```python
from build123d import *

# Parameters (mm, degrees)
F0_W      = 10
F0_H      = 79
F1_DEPTH  = 10
F2_W      = 10
F2_H      = 2
F3_DEPTH  = 15
F4_W      = 10
F4_H      = 2
F5_DEPTH  = 30
F7_DEPTH  = 10.001
F8_R      = 0.99999
F9_W      = 4.9229283333
F9_H      = 15
F10_DEPTH = 7


# Not quite as in the source:
# - a fillet or chamfer is up to 0.001 mm smaller than in the source, because OpenCascade refuses the exact size


with BuildPart() as f1:
    # F0 (on Top) → F1 (new body)
    with BuildSketch(Plane.XY):
        Rectangle(F0_W, F0_H)
    extrude(amount=F1_DEPTH)

    # F2 (on face) → F3 (join)
    with BuildSketch(Plane.XY.offset(10)):
        with Locations((0, -38.5)):
            Rectangle(F2_W, F2_H)
    extrude(amount=F3_DEPTH)

    # F4 (on face) → F5 (join)
    with BuildSketch(Plane.XY.offset(10)):
        with Locations((0, 38.5)):
            Rectangle(F4_W, F4_H)
    extrude(amount=F5_DEPTH)

    # F6 (on face) → F7 (cut, through all)
    with BuildSketch(Plane.YZ.offset(5)):
        Polygon((34.5, 5), (-43.3395786217, 0), (34.5, 0), align=None)
    extrude(amount=-F7_DEPTH, mode=Mode.SUBTRACT)

    # F8 (radius 1 in the source; OpenCascade refuses exactly that, so slightly less here)
    f8_edges = [f1.edges().sort_by_distance(p)[0] for p in [
        (0, -39.5, 25),
        (0, -37.5, 25),
        (0, 37.5, 40),
        (0, 39.5, 40),
        (0, -37.5, 10),
        (0, 37.5, 10),
    ]]
    fillet(f8_edges, radius=F8_R)

    # F9 (on face) → F10 (cut)
    with BuildSketch(Plane.YZ.offset(5)):
        with Locations((-37.0385358334, 17.5)):
            Rectangle(F9_W, F9_H)
    extrude(amount=-F10_DEPTH, mode=Mode.SUBTRACT)


solid = f1.part
```
Geometry check sheet. Reference: the model listing, model coordinates, mm. A direction names the side the tool comes from. Round coordinates to 2 decimals unless told otherwise and drop trailing zeros. Order: outer loops, then holes, each group sorted by start corner. A loop starts at its lowest first (then second) coordinate and runs counter-clockwise, first axis right, second up. Notation, with made-up numbers: (-40, 38) - (-12, 38) arc R20 cw to (-12, 69) - close; hole circle Ø3 at (-38.75, -25.75). An arc over 180 degrees is marked (long way). Use a Markdown table: item, result. Add a question column.
(1) Tool access check on faces 1 (the flat face through (-2, -39, 18)), 2 (the flat face through (0.07, -1.982, 2.657)), 3 (the flat face through (0, 37, 0)), 4 (the flat face through (0, 37.5, 25)), 5 (the flat face through (5, 2.7, 9.5)). Record the directions out of +Z, -Z, +X, -X, +Y, -Y that give a thin tool (end or side, any length) a straight path to the whole face; none if there is none.
(2) Sectioned sample at B-B, the plane z = 23. Enter the section's corners in (x, y).
(3) Release check for a two-part mould opening along Y. For faces 6 (the flat face through (0, 34.5, 2)), 7 (the flat face through (-4, -37.5, 17)), 8 (the flat face through (-5, -0.2, 9.5)), 9 (the flat face through (-1, -39.5, 9)) record: pulls with the +Y half, pulls with the -Y half, needs draft (parallel to the pull), parting line crosses it, or undercut.
(4) Material ranges on line 1 along Y through (x, z) = (-4.25, 13); line 2 along Y through (x, z) = (1.75, 37); line 3 along Z through (x, y) = (4.75, 35), recorded low to high. Write a range as [from, to].
(5) Depth check by flat-ended pin: pin 1 (6 mm diameter, centred on x = -1.5, y = -18.5, fed in from -Z); pin 2 (0.9 mm diameter, centred on y = -37.5, z = 18.5, fed in from +X); pin 3 (3 mm diameter, centred on x = 3.5, y = -1, fed in from -Z). Enter the tip coordinate at first touch or a pass-through.
(6) Sectioned sample at D-D, the plane z = 37. Enter the section's corners in (x, y), and give its area (3 significant figures).
Answers below:
| question | item | result |
|---|---|---|
| 1 | face 1 | +Z, +X, -Y |
| 1 | face 2 | -Z, +X, -X |
| 1 | face 3 | -Z, +X, -X, +Y, -Y |
| 1 | face 4 | +Z, +X, -X |
| 1 | face 5 | +Z, -Z, +X, +Y, -Y |
| 2 | outline | (-5, -39.5) - (-2, -39.5) - (-2, -37.5) - (-5, -37.5) - close; (-5, 37.5) - (5, 37.5) - (5, 39.5) - (-5, 39.5) - close |
| 3 | face 6 | undercut |
| 3 | face 7 | undercut |
| 3 | face 8 | needs draft |
| 3 | face 9 | pulls with the -Y half |
| 4 | line 1 | [-39.5, -37.5], [37.5, 39.5] |
| 4 | line 2 | [37.5, 39.5] |
| 4 | line 3 | [0, 10] |
| 5 | pin 1 | z = 1.4 |
| 5 | pin 2 | x = -2 |
| 5 | pin 3 | z = 2.62 |
| 6 | outline | (-5, 37.5) - (5, 37.5) - (5, 39.5) - (-5, 39.5) - close |
| 6 | area | 20.0 mm² |
